Geometry check sheet. Reference: the model listing, model coordinates, mm. Face numbers are marked on the shaded views. A direction names the side the tool comes from. Round coordinates to 2 decimals unless told otherwise and drop trailing zeros. Order: outer loops, then holes, each group sorted by start corner. A loop starts at its lowest first (then second) coordinate and runs counter-clockwise, first axis right, second up. Notation, with made-up numbers: (-17.5, -26.5) - (3.5, -26.5) arc R20 cw to (3.5, -21.5) - close; hole circle Ø6 at (-14, 38). An arc over 180 degrees is marked (long way). Write each question's results on one line, items separated by ' | '.
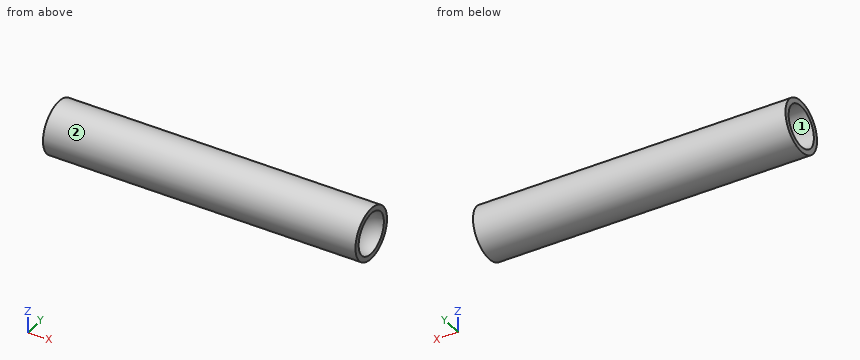
```python
from build123d import *

# Parameters (mm, degrees)
SKETCH1_R           = 25
BOSS_EXTRUDE1_DEPTH = 300
SKETCH3_R           = 20
CUT_EXTRUDE1_DEPTH  = 200


with BuildPart() as part:
    # Sketch1 → Boss-Extrude1 (new body)
    with BuildSketch(Plane(origin=(0, 0, 0), x_dir=(0, 0, -1), z_dir=(1, 0, 0))):
        Circle(SKETCH1_R)
    extrude(amount=BOSS_EXTRUDE1_DEPTH)

    # Sketch2 → Cut-Revolve3 (revolve, cut)
    with BuildSketch(Plane(origin=(300, 0, 0), x_dir=(0, 0, -1), z_dir=(1, 0, 0))):
        with BuildLine():
            Line((-20, 0), (20, 0))
            ThreePointArc((20, 0), (0, 20), (-20, 0))
        make_face()
    revolve(axis=Axis((300, 0, 20), (0, 0, -1)), mode=Mode.SUBTRACT)

    # Sketch3 → Cut-Extrude1 (cut)
    with BuildSketch(Plane.ZY):
        Circle(SKETCH3_R)
    extrude(amount=-CUT_EXTRUDE1_DEPTH, mode=Mode.SUBTRACT)


solid = part.part
```
(1) Depth check by flat-ended pin: pin 1 Ø3 at (x, z) = (54.5, -13) entering from -Y; pin 2 Ø3 at (x, y) = (252, -8) entering from -Z; pin 3 Ø3 at (x, y) = (160, -7) entering from -Z. Enter the tip coordinate at first touch or a pass-through.
Answers follow:
pin 1: y = -22.2 | pin 2: z = -24.14 | pin 3: z = -24.39
(2) Section check B-B (z = 16.5). Record the cut outline in (x, y).
Answers follow:
outline: (0, -18.78) - (300, -18.78) - (300, -11.3) arc R11.3 cw to (300, 11.3) - (300, 18.78) - (0, 18.78) - (0, 11.3) - (200, 11.3) - (200, -11.3) - (0, -11.3) - close
(3) Section check A-A (y = 0). Record the cut outline in (x, z), then the cut area to 3 significant figures.
Answers follow:
outline: (0, -25) - (300, -25) - (300, -20) arc R20 cw to (300, 20) - (300, 25) - (0, 25) - (0, 20) - (200, 20) - (200, -20) - (0, -20) - close | area: 6,370 mm²
(4) Section check C-C (x = 100). Record the cut outline in (y, z), then the cut area to 3 significant figures.
Answers follow:
outline: circle Ø50 at (0, 0); hole circle Ø40 at (0, 0) | area: 707 mm²
(5) Material ranges on line 1 (Y direction, x = 65, z = 0); line 2 (Z direction, x = 205.5, y = -1); line 3 (Z direction, x = 62.5, y = 5.5), recorded low to high.
Answers follow:
line 1: -25 to -20, 20 to 25 | line 2: -24.98 to 24.98 | line 3: -24.39 to -19.23, 19.23 to 24.39
(6) Access from +Z, -Z, +X, -X, +Y, -Y to the whole of each face (thin tool, end or side, straight path). Record for the marked faces 1 and 2.
Answers follow:
face 1: -X | face 2: +X, -X
